Design review of the part built by this model. Coordinates are the model's own, in mm. A direction names the side the tool comes from. Coordinates: 2 decimals unless noted, no trailing zeros. Write each loop counter-clockwise with the first axis right and the second up, starting at its lowest first coordinate (ties: lowest second). Pieces come first, ordered by that corner, then holes.
Q1. Clearance check with flat-ended pins moving along their axes: pin 1 Ø22.5 at (x, z) = (5.5, 0) entering from -Y; pin 2 Ø8 at (x, y) = (8.5, 139.5) entering from +Z; pin 3 Ø8 at (x, z) = (27, 20) entering from -Y. State where each tip first meets the part, or that it passes through.
Q2. Add section B-B, the plane y = 87. Give the boundary of the cut face in (x, z), plus the area to 3 significant figures.
Q3. The part is to be moulded in two halves that separate along Z. For faces 1 (the face through (11.26, 25.16, -35.77)), 2 (the face through (-39, 0, 0)), 3 (the face through (13.52, 23.6, 42.92)), 4 (the face through (-0.976, 32.436, 0.525)), say which applies: +Z half, -Z half, draft (parallel to the pull), parting line (faces both ways), or undercut.
Q4. To check wall thickness, follow probe 1 along X at (y, z) = (33.5, 0); probe 2 along X at (y, z) = (27, 0). State the ranges of each line that lie inside material, in increasing order.
Q5. Add section A-A, the plane y = 188. Give the boundary of the cut face in (x, z).
Q6. Machinability: for faces 5 (the face through (-14.99, 145.84, -19.54)), 6 (the face through (1, 50, -1)), which of the approach directions +Z, -Z, +X, -X, +Y, -Y give a long, thin tool a straight path to every point of the face, cutting with its end or side? Answer none if there is none.
from build123d import *

# Parameters (mm, degrees)
SKETCH_1_R          = 45
EXTRUDE_1_DEPTH     = 50
SKETCH_2_R          = 37.5
CUT_EXTRUDE_1_DEPTH = 50
SKETCH_3_R          = 7.5
EXTRUDE_2_DEPTH     = 80
SKETCH_4_R          = 45
EXTRUDE_3_DEPTH     = 190
EXTRUDE_3_TAPER     = 12
FILLET_1_R          = 5
FILLET_2_R          = 30
CHAMFER_1_SIZE      = 1


with BuildPart() as part:
    # 草图1 → 凸台-拉伸1 (new body)
    with BuildSketch(Plane(origin=(0, 0, 0), x_dir=(1, 0, 0), z_dir=(0, 1, 0))):
        with Locations(Location((0, 0, 0), (0, 0, 270))):
            Circle(SKETCH_1_R)
    extrude(amount=EXTRUDE_1_DEPTH)

    # 草图2 → 切除-拉伸1 (cut)
    with BuildSketch(Plane(origin=(0, 0, 0), x_dir=(-1, 0, 0), z_dir=(0, -1, 0))):
        with Locations(Location((0, 0, 0), (0, 0, 90))):
            Circle(SKETCH_2_R)
    extrude(amount=-CUT_EXTRUDE_1_DEPTH, mode=Mode.SUBTRACT)

    # 草图3 → 凸台-拉伸2 (add)
    with BuildSketch(Plane.XY.offset(40)):
        with Locations((0, 25)):
            Circle(SKETCH_3_R)
    extrude(amount=-EXTRUDE_2_DEPTH)

    # 草图4 → 凸台-拉伸3 (add)
    with BuildSketch(Plane(origin=(0, 50, 0), x_dir=(1, 0, 0), z_dir=(0, 1, 0))):
        with Locations(Location((0, 0, 0), (0, 0, 270))):
            Circle(SKETCH_4_R)
    extrude(amount=EXTRUDE_3_DEPTH, taper=EXTRUDE_3_TAPER)

    # 圆角1
    fillet_1_edges = [part.edges().sort_by_distance(p)[0] for p in [
        (0, 240, -4.614253283),
    ]]
    fillet(fillet_1_edges, radius=FILLET_1_R)

    # 圆角2
    fillet_2_edges = [part.edges().sort_by_distance(p)[0] for p in [
        (0, 50, -45),
    ]]
    fillet(fillet_2_edges, radius=FILLET_2_R)

    # 倒角1
    chamfer_1_edges = [part.edges().sort_by_distance(p)[0] for p in [
        (0, 0, -45),
        (0, 0, 37.5),
    ]]
    chamfer(chamfer_1_edges, length=CHAMFER_1_SIZE)


solid = part.part
Here are the results:
1. pin 1: stops at y = 17.5
1. pin 2: stops at z = 25.97
1. pin 3: stops at y = 0.9
2. outline: circle Ø74.27 at (0, 0)
2. area: 4,330 mm2
3. face 1: undercut
3. face 2: draft
3. face 3: parting line
3. face 4: undercut
4. probe 1: x = -45 to -37.5, 37.5 to 45
4. probe 2: x = -45 to -37.5, -7.23 to 7.23, 37.5 to 45
5. outline: circle Ø31.33 at (0, 0)
6. face 5: +Y
6. face 6: none
